For this review, take the finished solid that the model builds, in its own axes (mm). Face numbers are marked on the shaded views. A direction names the side the tool comes from. Coordinates: 2 decimals unless noted, no trailing zeros. Loops run counter-clockwise (first coordinate to the right, second up) from the corner with the lowest first, then second, coordinate; pieces in that order, holes last.
1. To check wall thickness, follow probe 1 along Y at (x, z) = (-5.25, -6.75); probe 2 along X at (y, z) = (4.5, 4.5); probe 3 along X at (y, z) = (2.75, 5). State the ranges of each line that lie inside material, in increasing order.
2. Take a section at C-C, the plane z = -3.75. State the section outline as (x, y) points, then the cut area to 3 significant figures.
3. Machinability: for the marked faces 1, 2 and 3, which of the approach directions +Z, -Z, +X, -X, +Y, -Y give a long, thin tool a straight path to every point of the face, cutting with its end or side? Answer none if there is none.
4. Take a section at A-A, the plane y = 1.25. State the section outline as (x, z) points, then the cut area to 3 significant figures.
5. Take a section at D-D, the plane y = 7.25. State the section outline as (x, z) points, then the cut area to 3 significant figures.
6. Clearance check with flat-ended pins moving along their axes: P1, Ø1.5, axis at x = -5.5, y = 2.5, coming from the +Z side; P2, Ø1.5, axis at y = 4, z = -1, coming from the +X side; P3, Ø1, axis at y = 5.5, z = 2.5, coming from the +X side; P4, Ø4, axis at y = 11, z = -4, coming from the -X side. State where each tip first meets the part, or that it passes through.
7. Take a section at B-B, the plane x = 1. State the section outline as (y, z) points, then the cut area to 3 significant figures.
```python
from build123d import *

# Parameters (mm, degrees)
SKETCH_1_R          = 10
EXTRUDE_1_DEPTH     = 7
SKETCH_2_R          = 1.7
EXTRUDE_2_DEPTH     = 5
CUT_EXTRUDE_1_DEPTH = 7


with BuildPart() as part:
    # 草图1 → 凸台-拉伸1 (new body)
    with BuildSketch(Plane(origin=(0, 0, 0), x_dir=(1, 0, 0), z_dir=(0, 1, 0))):
        with Locations(Location((0, 0, 0), (0, 0, 270))):
            Circle(SKETCH_1_R)
    extrude(amount=EXTRUDE_1_DEPTH)

    # 草图2 → 凸台-拉伸2 (add)
    with BuildSketch(Plane(origin=(0, 7, 0), x_dir=(1, 0, 0), z_dir=(0, 1, 0))):
        with BuildLine():
            ThreePointArc((6.618999669, 0.253451944), (6.623850429, 0), (6.618999669, -0.253451944))
            ThreePointArc((6.618999669, -0.253451944), (10, 0), (6.618999669, 0.253451944))
        make_face()
        with Locations(Location((0, 8.3, 0), (0, 0, 89.999317856))):
            Circle(SKETCH_2_R)
        with Locations(Location((0, -8.3, 0), (0, 0, 269.999317859))):
            Circle(SKETCH_2_R)
        with Locations(Location((-8.3, 0, 0), (0, 0, 179.999317857))):
            Circle(SKETCH_2_R)
    extrude(amount=EXTRUDE_2_DEPTH)

    # 草图3 → 切除-拉伸1 (cut)
    with BuildSketch(Plane(origin=(0, 7, 0), x_dir=(1, 0, 0), z_dir=(0, 1, 0))):
        Polygon((-5.581963916, 3.029028256), (-5.414197376, -3.319608426), (0.16776654, -6.348636682), (5.581963916, -3.029028256), (5.414197376, 3.319608426), (-0.16776654, 6.348636682), align=None)
    extrude(amount=-CUT_EXTRUDE_1_DEPTH, mode=Mode.SUBTRACT)


solid = part.part
```
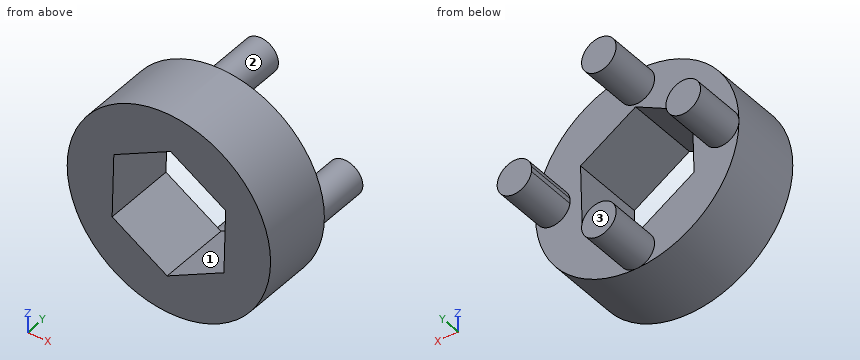
Results list:
1. probe 1: y = 0 to 7
1. probe 2: x = -8.93 to -3.24, 3.18 to 8.93
1. probe 3: x = -8.66 to -2.32, 2.37 to 8.66
2. outline: (-9.27, 0) - (-4.41, 0) - (-4.41, 7) - (-9.27, 7) - close; (4.62, 0) - (9.27, 0) - (9.27, 7) - (4.62, 7) - close
2. area: 66.6 mm2
3. face 1: +Y, -Y
3. face 2: +Y
3. face 3: +Z, -Z, +X, -X, +Y
4. outline: circle Ø20 at (0, 0); hole (-5.58, -3.03) - (-0.17, -6.35) - (5.41, -3.32) - (5.58, 3.03) - (0.17, 6.35) - (-5.41, 3.32) - close
4. area: 209 mm2
5. outline: circle Ø3.4 at (-8.3, 0); circle Ø3.4 at (0, -8.3); circle Ø3.4 at (0, 8.3); (6.62, -0.25) arc R1.7 ccw (long way) to (6.62, 0.25) arc R6.62 cw to start
5. area: 36.3 mm2
6. P1: stops at z = 8.8
6. P2: stops at x = 10
6. P3: stops at x = 9.8
6. P4: passes through
7. outline: (0, -9.95) - (7, -9.95) - (7, -9.67) - (12, -9.67) - (12, -6.93) - (7, -6.93) - (7, -5.71) - (0, -5.71) - close; (0, 5.84) - (7, 5.84) - (7, 6.93) - (12, 6.93) - (12, 9.67) - (7, 9.67) - (7, 9.95) - (0, 9.95) - close
7. area: 85.9 mm2
